The model under review builds one solid part; all positions refer to its coordinate system, in mm. Coordinates: 2 decimals unless noted, no trailing zeros. Order: outer loops, then holes, each group sorted by start corner. A loop starts at its lowest first (then second) coordinate and runs counter-clockwise, first axis right, second up. Notation, with made-up numbers: M 41,87.5 L 68,87.5 A13 ccw 68,92.5 Z; hole C 50.5,20 d7. An arc over 180 degrees is marked long. Write each question's results on one line, items separated by ' | '.
from build123d import *

# Parameters (mm, degrees)
SKETCH1_W           = 200.5584
SKETCH1_H           = 162.3568
BOSS_EXTRUDE1_DEPTH = 7.2136
SKETCH2_W           = 7.2136
SKETCH2_H           = 18.4912
SKETCH2_W_2         = 20.05584
SKETCH2_H_2         = 7.2136
SKETCH2_W_3         = 40.11168
CUT_EXTRUDE1_DEPTH  = 200.347884659


with BuildPart() as part:
    # Sketch1 → Boss-Extrude1 (new body)
    with BuildSketch(Plane(origin=(0, 0, 0), x_dir=(1, 0, 0), z_dir=(0, 1, 0))):
        with Locations((54.486535415, -44.261267707)):
            Rectangle(SKETCH1_W, SKETCH1_H)
    extrude(amount=BOSS_EXTRUDE1_DEPTH)

    # Sketch2 → Cut-Extrude1 (cut, through all)
    with BuildSketch(Plane(origin=(0, 7.2136, 0), x_dir=(1, 0, 0), z_dir=(0, 1, 0))):
        with Locations((-42.185864585, -71.998067707)):
            Rectangle(SKETCH2_W, SKETCH2_H)
        with Locations((-42.185864585, -108.980467707)):
            Rectangle(SKETCH2_W, SKETCH2_H)
        Polygon((-45.792664585, -125.439667707), (-5.680984585, -125.439667707), (-5.680984585, -118.226067707), (-38.579064585, -118.226067707), (-45.792664585, -118.226067707), align=None)
        with Locations((64.514455415, -121.832867707)):
            Rectangle(SKETCH2_W_2, SKETCH2_H_2)
        with Locations((44.458615415, -121.832867707)):
            Rectangle(SKETCH2_W_2, SKETCH2_H_2)
        with Locations((134.709895415, -121.832867707)):
            Rectangle(SKETCH2_W_3, SKETCH2_H_2)
        with Locations((151.158935415, -108.980467707)):
            Rectangle(SKETCH2_W, SKETCH2_H)
        with Locations((151.158935415, -71.998067707)):
            Rectangle(SKETCH2_W, SKETCH2_H)
        with Locations((151.158935415, -16.524467707)):
            Rectangle(SKETCH2_W, SKETCH2_H)
        with Locations((151.158935415, 20.457932293)):
            Rectangle(SKETCH2_W, SKETCH2_H)
        with Locations((134.709895415, 33.310332293)):
            Rectangle(SKETCH2_W_3, SKETCH2_H_2)
        with Locations((54.486535415, 33.310332293)):
            Rectangle(SKETCH2_W_3, SKETCH2_H_2)
        with Locations((-42.185864585, -16.524467707)):
            Rectangle(SKETCH2_W, SKETCH2_H)
        with Locations((-42.185864585, 20.457932293)):
            Rectangle(SKETCH2_W, SKETCH2_H)
        with Locations((-25.736824585, 33.310332293)):
            Rectangle(SKETCH2_W_3, SKETCH2_H_2)
    extrude(amount=-CUT_EXTRUDE1_DEPTH, mode=Mode.SUBTRACT)


solid = part.part
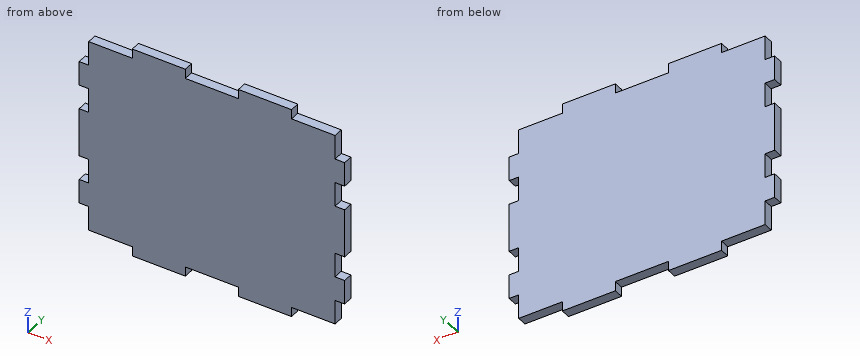
1) Take a section at A-A on x = -11. State the section outline as (y, z) points, plus the area to 3 significant figures.
Solutions:
outline: M 0,-29.7 L 7.21,-29.7 L 7.21,118.23 L 0,118.23 Z | area: 1,070 mm2
2) For pin 1 (2 mm diameter, centred on x = 152, y = 3.5, fed in from +Z); pin 2 (3.5 mm diameter, centred on y = 2, z = 122, fed in from -X); pin 3 (2 mm diameter, centred on x = 151, y = 4, fed in from -Z), all flat-tipped, find the tip position at first contact; note any pin that passes through.
Solutions:
pin 1: z = 99.73 | pin 2: x = -5.68 | pin 3: z = -11.21
3) Take a section at B-B on z = -21. State the section outline as (x, y) points, plus the area to 3 significant figures.
Solutions:
outline: M -38.58,0 L 147.55,0 L 147.55,7.21 L -38.58,7.21 Z | area: 1,340 mm2
4) To check wall thickness, follow line 1 along X through (y, z) = (3.75, 16); line 2 along Z through (x, y) = (-23.5, 3). State the ranges of each line that lie inside material, in increasing order.
Solutions:
line 1: -38.58 to 147.55 | line 2: -29.7 to 118.23
